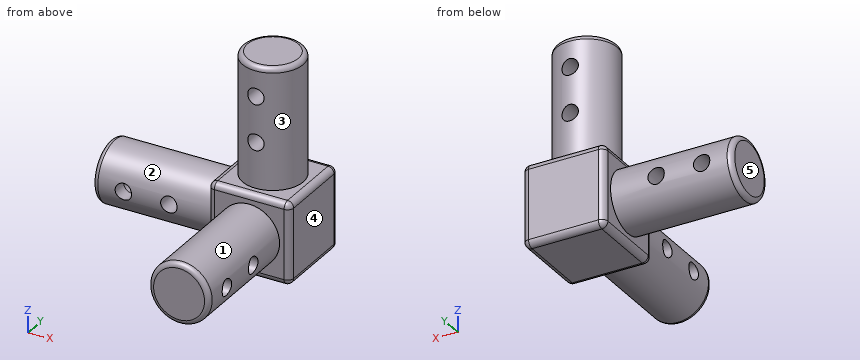
```python
from build123d import *

# Parameters (mm, degrees)
F0_W      = 34.29
F0_H      = 34.29
F1_DEPTH  = 34.29
F2_R      = 12.7
F3_DEPTH  = 50.8
F4_R      = 12.7
F5_DEPTH  = 50.8
F6_R      = 12.7
F7_DEPTH  = 50.8
F8_R      = 3.429
F9_DEPTH  = 25.4
F10_R     = 3.429
F11_DEPTH = 25.4
F12_R     = 3.429
F13_DEPTH = 25.4
F14_R     = 2.032
F15_R     = 2.54


with BuildPart() as f1:
    # F0 (on Top) → F1 (new body)
    with BuildSketch(Plane.XY):
        with Locations((3.672889, 6.561064)):
            Rectangle(F0_W, F0_H)
    extrude(amount=F1_DEPTH)

    # F2 (on face) → F3 (join)
    with BuildSketch(Plane.XY.offset(34.29)):
        with Locations((3.682848, 6.561064)):
            Circle(F2_R)
    extrude(amount=F3_DEPTH)

    # F4 (on face) → F5 (join)
    with BuildSketch(Plane(origin=(-13.472111, 0, 0), x_dir=(0, -1, 0), z_dir=(-1, 0, 0))):
        with Locations((-6.561064, 17.145)):
            Circle(F4_R)
    extrude(amount=F5_DEPTH)

    # F6 (on face) → F7 (join)
    with BuildSketch(Plane.XZ.offset(10.583936)):
        with Locations((3.672889, 17.145)):
            Circle(F6_R)
    extrude(amount=F7_DEPTH)

    # F8 (on Front) → F9 (cut, symmetric)
    with BuildSketch(Plane.XZ):
        with Locations((3.672889, 53.34)):
            Circle(F8_R)
        with Locations((3.672889, 72.39)):
            Circle(F8_R)
    extrude(amount=F9_DEPTH, both=True, mode=Mode.SUBTRACT)

    # F10 (on Right) → F11 (cut, symmetric)
    with BuildSketch(Plane.YZ):
        with Locations((-29.633936, 17.145)):
            Circle(F10_R)
        with Locations((-48.683936, 17.145)):
            Circle(F10_R)
    extrude(amount=F11_DEPTH, both=True, mode=Mode.SUBTRACT)

    # F12 (on Front) → F13 (cut, symmetric)
    with BuildSketch(Plane.XZ):
        with Locations((-51.572111, 17.145)):
            Circle(F12_R)
        with Locations((-32.522111, 17.145)):
            Circle(F12_R)
    extrude(amount=F13_DEPTH, both=True, mode=Mode.SUBTRACT)

    # F14
    f14_edges = [f1.edges().sort_by_distance(p)[0] for p in [
        (-9.017152, 6.561064, 85.09),
        (-9.027111, -61.383936, 17.145),
        (-64.272111, 19.261064, 17.145),
    ]]
    fillet(f14_edges, radius=F14_R)

    # F15
    f15_edges = [f1.edges().sort_by_distance(p)[0] for p in [
        (20.817889, 23.706064, 17.145),
        (20.817889, 6.561064, 34.29),
        (20.817889, -10.583936, 17.145),
        (20.817889, 6.561064, 0),
        (3.672889, 23.706064, 0),
        (3.672889, 23.706064, 34.29),
        (-13.472111, 23.706064, 17.145),
        (-13.472111, 6.561064, 0),
        (3.672889, -10.583936, 0),
        (-13.472111, 6.561064, 34.29),
        (-13.472111, -10.583936, 17.145),
        (3.672889, -10.583936, 34.29),
    ]]
    fillet(f15_edges, radius=F15_R)


solid = f1.part
```
Model file for the job. Use its own axes, mm. Face numbers are marked on the shaded views. A direction names the side the tool comes from. Coordinates: 2 decimals unless noted, no trailing zeros. Order: outer loops, then holes, each group sorted by start corner. A loop starts at its lowest first (then second) coordinate and runs counter-clockwise, first axis right, second up. Notation, with made-up numbers: (-2.5, -30.5) - (26.5, -30.5) arc R12 ccw to (26.5, -21.5) - close; hole circle Ø4 at (48, -1.5). An arc over 180 degrees is marked (long way). Return JSON: item names as keys, results as strings. Group by question number.
1) Saw through at A-A, the plane y = -47. Write the cut outline in (x, z) (3 decimals), plus the area to 3 significant figures.
2) Saw through at B-B, the plane z = 55. Write the cut outline in (x, y).
3) Saw through at D-D, the plane y = -18.5. Write the cut outline in (x, z) (3 decimals).
4) Probe line 1 (Y direction, x = -57.5, z = 24); line 2 (X direction, y = 7, z = 73.5); line 3 (Z direction, x = -7, y = -3). List the from-to ranges inside material, lowest first. Write a range as from..to.
5) Tool access for the marked faces 1, 2, 3, 4 and 5: list every direction of +Z, -Z, +X, -X, +Y, -Y with a clear straight run to the whole face (end or side of a thin tool).
6) Saw through at C-C, the plane x = -1.5. Count the separate pieces of the cut face and the enclosed holes in it, plus the area to 3 significant figures.
7) Flat gauge pins, fed straight in: P1, Ø9, axis at y = -29.63, z = 17.14, coming from the -X side; P2, Ø12, axis at y = -16.5, z = 66.5, coming from the +X side; P3, Ø9, axis at y = -48.68, z = 17.14, coming from the +X side; P4, Ø3, axis at y = -11.5, z = 20.5, coming from the +X side. Where does each tip first touch, or does it go through?
Values found:
{
 "1": {"outline": "(-8.671, 14.158) arc R12.7 ccw to (16.017, 14.158) - close; (-8.671, 20.132) - (16.017, 20.132) arc R12.7 ccw to start", "area": "356 mm²"},
 "2": {"outline": "(0.67, -5.78) - (0.67, 18.9) arc R12.7 ccw to start; (6.67, -5.78) arc R12.7 ccw to (6.67, 18.9) - close"},
 "3": {"outline": "circle Ø25.4 at (3.673, 17.145)"},
 "4": {"line 1": "y = -4.13..17.25", "line 2": "x = -9.01..0.43, 6.92..16.38", "line 3": "z = 0..34.29"},
 "5": {"face 1": "-Y", "face 2": "-X", "face 3": "+Z", "face 4": "+Z, -Z, +X, +Y, -Y", "face 5": "+Z, -Z, -X, +Y, -Y"},
 "6": {"separate pieces": "1", "enclosed holes": "2", "area": "3,450 mm²"},
 "7": {"P1": "stops at x = -9.03", "P2": "passes through", "P3": "stops at x = 16.37", "P4": "stops at x = 19.9"}
}
